```python
from build123d import *

# Parameters (mm, degrees)
BOSS_EXTRUDE1_DEPTH                  = 6.35
CUT_EXTRUDE1_REACH                   = 8.35
SKETCH2_R                            = 3.3782
F_3_8_CLEARANCE_HOLE1_D              = 9.8044
F_3_8_CLEARANCE_HOLE1_CSINK_D        = 11.58748
F_3_8_CLEARANCE_HOLE1_CSINK_ANGLE    = 90
F_1_4_0_2500_DOWEL_HOLE1_D           = 6.35
F_1_4_0_2500_DOWEL_HOLE1_CSINK_D     = 7.62
F_1_4_0_2500_DOWEL_HOLE1_CSINK_ANGLE = 90
CUT_EXTRUDE2_DEPTH                   = 7.35


with BuildPart() as part:
    # Sketch1 → Boss-Extrude1 (new body)
    with BuildSketch(Plane(origin=(0, 0, 0), x_dir=(0, 0, -1), z_dir=(1, 0, 0))):
        with BuildLine():
            Line((-74.539032088, -105.353687095), (-11.039032088, 6.279312905))
            ThreePointArc((-11.039032088, 6.279312905), (-1.199563995, 12.643221355), (9.661154553, 8.243305933))
            Line((9.661154553, 8.243305933), (104.911154553, -103.389694067))
            ThreePointArc((104.911154553, -103.389694067), (106.782128714, -116.95277512), (95.25, -124.333))
            Line((95.25, -124.333), (-63.5, -124.333))
            ThreePointArc((-63.5, -124.333), (-74.478098057, -118.018245731), (-74.539032088, -105.353687095))
        make_face()
    extrude(amount=BOSS_EXTRUDE1_DEPTH)

    # Sketch2 → Cut-Extrude1 (cut, up to next)
    with BuildSketch(Plane(origin=(6.35, 0, 0), x_dir=(0, 0, -1), z_dir=(1, 0, 0)), mode=Mode.PRIVATE) as cut_extrude1_sk1:
        with Locations((-63.5, -111.633)):
            Circle(SKETCH2_R)
    cut_extrude1_tool1 = extrude(cut_extrude1_sk1.sketch, amount=-CUT_EXTRUDE1_REACH, mode=Mode.PRIVATE) & part.part
    add(cut_extrude1_tool1.solids().sort_by_distance((6.35, -111.633, 63.5))[0], mode=Mode.SUBTRACT)
    # Sketch2 → Cut-Extrude1 (cut, up to next)
    with BuildSketch(Plane(origin=(6.35, 0, 0), x_dir=(0, 0, -1), z_dir=(1, 0, 0)), mode=Mode.PRIVATE) as cut_extrude1_sk2:
        with Locations((0, -111.633)):
            Circle(SKETCH2_R)
    cut_extrude1_tool2 = extrude(cut_extrude1_sk2.sketch, amount=-CUT_EXTRUDE1_REACH, mode=Mode.PRIVATE) & part.part
    add(cut_extrude1_tool2.solids().sort_by_distance((6.35, -111.633, 0))[0], mode=Mode.SUBTRACT)
    # Sketch2 → Cut-Extrude1 (cut, up to next)
    with BuildSketch(Plane(origin=(6.35, 0, 0), x_dir=(0, 0, -1), z_dir=(1, 0, 0)), mode=Mode.PRIVATE) as cut_extrude1_sk3:
        with Locations((95.25, -111.633)):
            Circle(SKETCH2_R)
    cut_extrude1_tool3 = extrude(cut_extrude1_sk3.sketch, amount=-CUT_EXTRUDE1_REACH, mode=Mode.PRIVATE) & part.part
    add(cut_extrude1_tool3.solids().sort_by_distance((6.35, -111.633, -95.25))[0], mode=Mode.SUBTRACT)

    # 3/8 Clearance Hole1 (through all)
    with Locations(Plane(origin=(6.35, 0, 0), x_dir=(0, 0, -1), z_dir=(1, 0, 0))):
        with Locations((0, 0)):
            CounterSinkHole(F_3_8_CLEARANCE_HOLE1_D / 2, F_3_8_CLEARANCE_HOLE1_CSINK_D / 2, counter_sink_angle=F_3_8_CLEARANCE_HOLE1_CSINK_ANGLE)

    # 1/4 (0.2500) Dowel Hole1 (through all)
    with Locations(Plane(origin=(6.35, 0, 0), x_dir=(0, 0, -1), z_dir=(1, 0, 0))):
        with Locations((-38.134262993, -79.883)):
            CounterSinkHole(F_1_4_0_2500_DOWEL_HOLE1_D / 2, F_1_4_0_2500_DOWEL_HOLE1_CSINK_D / 2, counter_sink_angle=F_1_4_0_2500_DOWEL_HOLE1_CSINK_ANGLE)

    # Sketch7 → Cut-Extrude2 (cut, through all)
    with BuildSketch(Plane(origin=(6.35, 0, 0), x_dir=(0, 0, -1), z_dir=(1, 0, 0))):
        with BuildLine():
            Line((-7.560548241, -21.370623035), (-23.109121722, -73.87283281))
            ThreePointArc((-23.109121722, -73.87283281), (-20.480108275, -81.000798522), (-12.898859563, -80.506556809))
            Line((-12.898859563, -80.506556809), (29.486651444, -44.341445027))
            ThreePointArc((29.486651444, -44.341445027), (31.69518119, -40.012152938), (30.195575755, -35.389214784))
            Line((30.195575755, -35.389214784), (14.277824698, -16.733610546))
            ThreePointArc((14.277824698, -16.733610546), (1.978846134, -12.553878022), (-7.560548241, -21.370623035))
        make_face()
        with BuildLine():
            Line((-2.594727147, -98.933), (56.882953013, -98.933))
            ThreePointArc((56.882953013, -98.933), (68.415081727, -91.55277512), (66.544107566, -77.989694067))
            Line((66.544107566, -77.989694067), (44.621361137, -52.296235252))
            ThreePointArc((44.621361137, -52.296235252), (40.292069047, -50.087705507), (35.669130894, -51.587310942))
            Line((35.669130894, -51.587310942), (-6.716380114, -87.752422723))
            ThreePointArc((-6.716380114, -87.752422723), (-8.552774886, -94.779398677), (-2.594727147, -98.933))
        make_face()
    extrude(amount=-CUT_EXTRUDE2_DEPTH, mode=Mode.SUBTRACT)


solid = part.part
```
The listing builds one solid part. Answer for the finished solid, in the listing's coordinates (mm). A direction names the side the tool comes from. Round coordinates to 2 decimals unless told otherwise and drop trailing zeros. Write each loop counter-clockwise with the first axis right and the second up, starting at its lowest first coordinate (ties: lowest second). Pieces come first, ordered by that corner, then holes. Notation, with made-up numbers: (2.25, 27.25) -> (29.25, 27.25) arc R26 cw to (29.25, 66.25) -> close; hole circle Ø11 at (52.25, 70). An arc over 180 degrees is marked (long way). Use CSV: the item, a comma, the result in double quotes. Start each with the question number.
(1) Each of these flat-tipped pins is pushed along its axis until it touches: pin 1 (4 mm diameter, centred on y = -100, z = -47, fed in from -X); pin 2 (1 mm diameter, centred on x = 3.5, y = -102, fed in from -Z); pin 3 (2 mm diameter, centred on x = 5, z = 42, fed in from +Y); pin 4 (4 mm diameter, centred on y = -79.88, z = 38.13, fed in from +X). Where does it stop, or does it pass through?
(2) Section D-D on z = -62 is taken. Give the vertices of the cut face in (x, y), then the cut area to 3 significant figures.
(3) Section A-A on y = -68 is taken. Give the vertices of the cut face in (x, z).
(4) Consider L1, parallel to Z at x = 6, y = -81; L2, parallel to Y at x = 6.25, z = -26; L3, parallel to Z at x = 6.25, y = -70. Determine where each line is inside the solid, lowest interval first. Write a range as from..to.
(5) Section B-B on z = -17.5 is taken. Give the vertices of the cut face in (x, y).
(6) Section C-C on y = -96 is taken. Give the vertices of the cut face in (x, z).
(7) Which of the six approach directions +Z, -Z, +X, -X, +Y, -Y give full straight-line access (tool end or side, diameter ignored) to faces 4 (the face through (3, -98.933, -27)), 5 (the face through (3.131, -116.768, -106.865))?
(8) The mould has two halves that part along Z. Classify faces 1 (the face through (3.131, 12.626, 1.369)), 2 (the face through (3.131, -50.319, 43.234)), 3 (the face through (3.22, -114.63, 61.94)): released by +Z, released by -Z, zero draft, split by the parting line, or undercut.
A:
1,pin 1,"stops at x = 0"
1,pin 2,"stops at z = -104.15"
1,pin 3,"stops at y = -46.39"
1,pin 4,"passes through"
2,outline,"(0, -124.33) -> (6.35, -124.33) -> (6.35, -97.86) -> (0, -97.86) -> close; (0, -72.66) -> (6.35, -72.66) -> (6.35, -53.1) -> (0, -53.1) -> close"
2,area,"292 mm²"
3,outline,"(0, -74.72) -> (6.35, -74.72) -> (6.35, -58.02) -> (0, -58.02) -> close; (0, -16.43) -> (6.35, -16.43) -> (6.35, -1.76) -> (0, -1.76) -> close; (0, 21.37) -> (6.35, 21.37) -> (6.35, 53.29) -> (0, 53.29) -> close"
4,L1,"z = -85.81..-68.45, -1.2..13.56, 20.48..34.86, 41.41..60.69"
4,L2,"y = -124.33..-98.93, -59.84..-47.32, -30.47..-10.91"
4,L3,"z = -76.42..-59.73, -14.09..0.59, 21.96..54.43"
5,outline,"(0, -124.33) -> (6.35, -124.33) -> (6.35, -98.93) -> (0, -98.93) -> close; (0, -67.09) -> (6.35, -67.09) -> (6.35, -54.57) -> (0, -54.57) -> close; (0, -20.51) -> (6.35, -20.51) -> (6.35, -0.94) -> (0, -0.94) -> close"
6,outline,"(0, -98.61) -> (6.35, -98.61) -> (6.35, -65) -> (0, -65) -> close; (0, 7.95) -> (6.35, 7.95) -> (6.35, 69.22) -> (0, 69.22) -> close"
7,face 4,"+X, -X"
7,face 5,"-Z, +X, -X"
8,face 1,"split by the parting line"
8,face 2,"released by +Z"
8,face 3,"undercut"
